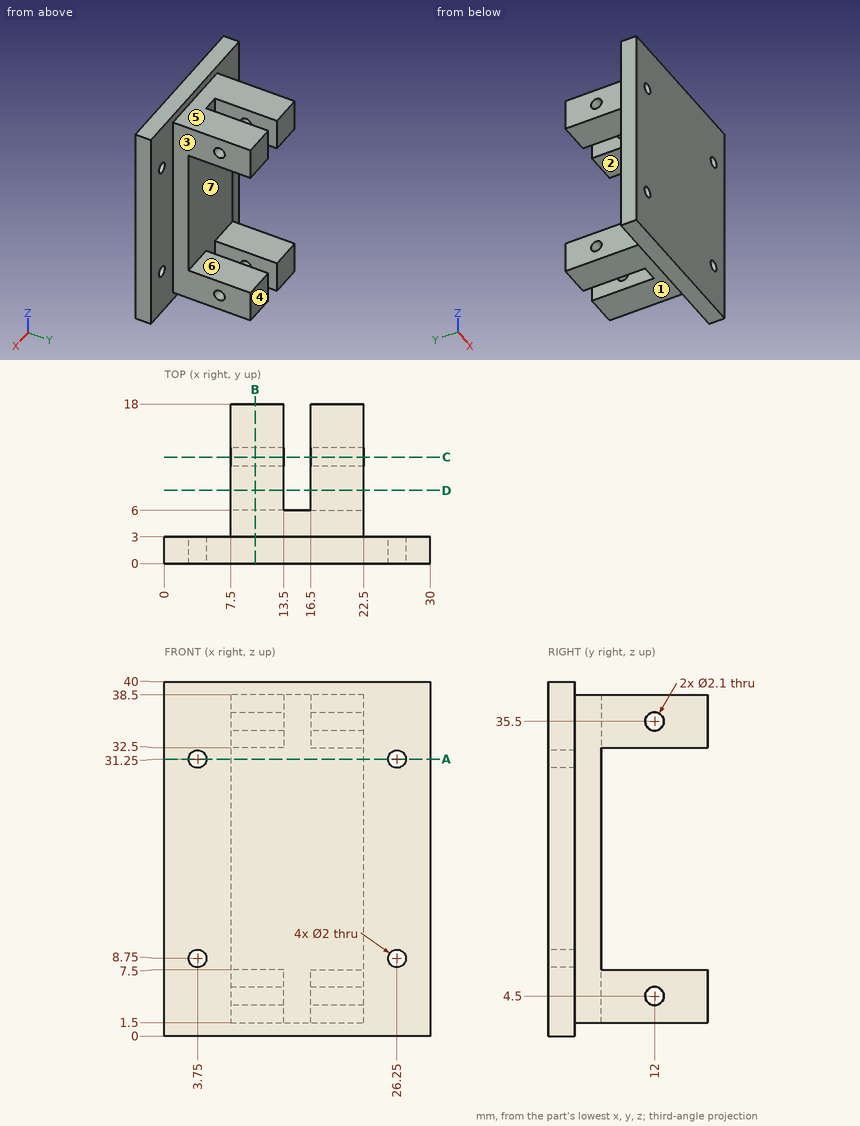
Part print with two shaded views. Sizes in mm from the minimum x, y, z corner. A direction names the side the tool comes from. Coordinates: 2 decimals unless noted, no trailing zeros. Write each loop counter-clockwise with the first axis right and the second up, starting at its lowest first coordinate (ties: lowest second). Pieces come first, ordered by that corner, then holes. Notation, with made-up numbers: (12, -25) - (19, -25) arc R28 cw to (19, 11) - close; hole circle Ø9 at (-20.75, 84). An arc over 180 degrees is marked (long way). Use a Markdown table: item, result. Add a question column.
Item 1: Drill centre lines: line 1 along Z through (x, y) = (26.25, 1.7); line 2 along Z through (x, y) = (10.3, 12); line 3 along X through (y, z) = (8, 33.5). Where is each one in solid material? Low to high.
Item 2: Drop flat-ended pins along their axis: pin 1 (7.5 mm diameter, centred on x = 13.5, y = 12.5, fed in from +Z); pin 2 (3 mm diameter, centred on x = 9.5, y = 14, fed in from -Z); pin 3 (5 mm diameter, centred on y = 13.5, z = 37, fed in from +X); pin 4 (1.2 mm diameter, centred on x = 3.75, z = 31.25, fed in from -Y). Give the stop position or say it passes through.
Item 3: 3-axis set-ups, long thin cutter, end or side, ignore diameter. For the marked faces 1, 2 and 3: which of +Z, -Z, +X, -X, +Y, -Y reach the whole face in a straight line?
Item 4: Band-saw the part on A-A, the plane z = 31.25. Write the cut outline in (x, y), and give its area (3 significant figures).
Item 5: Two-plate mould, pull along Z, no slides. Class the marked faces 4, 5, 6 and 7: pulls with the +Z half, pulls with the -Z half, needs draft (parallel to the pull), parting line crosses it, or undercut.
Item 6: Band-saw the part on C-C, the plane y = 12. Give the number of separate pieces and of enclosed holes in the cut face, and give its area (3 significant figures).
Item 7: Band-saw the part on D-D, the plane y = 8.25. Write the cut outline in (x, z), and give its area (3 significant figures).
Item 8: Band-saw the part on B-B, the plane x = 10.25. Write the cut outline in (y, z), and give its area (3 significant figures).
A:
| question | item | result |
|---|---|---|
| 1 | line 1 | z = 0 to 7.75, 9.75 to 30.25, 32.25 to 40 |
| 1 | line 2 | z = 1.5 to 3.45, 5.55 to 7.5, 32.5 to 34.45, 36.55 to 38.5 |
| 1 | line 3 | x = 7.5 to 13.5, 16.5 to 22.5 |
| 2 | pin 1 | stops at z = 38.5 |
| 2 | pin 2 | stops at z = 1.5 |
| 2 | pin 3 | stops at x = 22.5 |
| 2 | pin 4 | passes through |
| 3 | face 1 | -Z, +X, -X, +Y |
| 3 | face 2 | +X, -X, +Y |
| 3 | face 3 | +Z, -Z, +X, +Y |
| 4 | outline | (0, 0) - (2.75, 0) - (2.75, 3) - (0, 3) - close; (4.75, 0) - (25.25, 0) - (25.25, 3) - (22.5, 3) - (22.5, 6) - (7.5, 6) - (7.5, 3) - (4.75, 3) - close; (27.25, 0) - (30, 0) - (30, 3) - (27.25, 3) - close |
| 4 | area | 123 mm² |
| 5 | face 4 | needs draft |
| 5 | face 5 | pulls with the +Z half |
| 5 | face 6 | undercut |
| 5 | face 7 | undercut |
| 6 | separate pieces | 8 |
| 6 | enclosed holes | 0 |
| 6 | area | 93.6 mm² |
| 7 | outline | (7.5, 1.5) - (13.5, 1.5) - (13.5, 7.5) - (7.5, 7.5) - close; (7.5, 32.5) - (13.5, 32.5) - (13.5, 38.5) - (7.5, 38.5) - close; (16.5, 1.5) - (22.5, 1.5) - (22.5, 7.5) - (16.5, 7.5) - close; (16.5, 32.5) - (22.5, 32.5) - (22.5, 38.5) - (16.5, 38.5) - close |
| 7 | area | 144 mm² |
| 8 | outline | (0, 0) - (3, 0) - (3, 1.5) - (18, 1.5) - (18, 7.5) - (6, 7.5) - (6, 32.5) - (18, 32.5) - (18, 38.5) - (3, 38.5) - (3, 40) - (0, 40) - close; hole circle Ø2.1 at (12, 4.5); hole circle Ø2.1 at (12, 35.5) |
| 8 | area | 368 mm² |
